from build123d import *

# Parameters (mm, degrees)
SKETCH_1_W                      = 10
SKETCH_1_H                      = 4
EXTRUDE_1_DEPTH                 = 0.6
SKETCH_2_W                      = 6
SKETCH_2_H                      = 2.8
EXTRUDE_2_DEPTH                 = 2.5
FILLET_1_R                      = 1
CUT_EXTRUDE_2_REACH             = 9.134
SKETCH_7_W                      = 0.8
SKETCH_7_H                      = 1
CUT_EXTRUDE_2_DIRECTION_2_DEPTH = 8.134379197
SKETCH_8_W                      = 3.913502977
SKETCH_8_H                      = 4
EXTRUDE_3_DEPTH                 = 0.3
CUT_EXTRUDE_3_REACH             = 9.439
SKETCH_9_W                      = 2
SKETCH_9_H                      = 1
CHAMFER_2_SIZE                  = 0.6
FILLET_2_R                      = 0.3
SKETCH_10_W                     = 0.979037501
SKETCH_10_H                     = 2.8
SKETCH_10_W_2                   = 0.934465476
EXTRUDE_4_DEPTH                 = 1
CHAMFER_3_SIZE                  = 0.3


with BuildPart() as part:
    # 草图1 → 凸台-拉伸1 (new body)
    with BuildSketch(Plane(origin=(0, 0, 0), x_dir=(1, 0, 0), z_dir=(0, 1, 0))):
        with Locations((0.452464262, 0)):
            Rectangle(SKETCH_1_W, SKETCH_1_H)
    extrude(amount=EXTRUDE_1_DEPTH)

    # 草图2 → 凸台-拉伸2 (add)
    with BuildSketch(Plane(origin=(0, 0.6, 0), x_dir=(1, 0, 0), z_dir=(0, 1, 0))):
        with Locations((0.452464262, 0)):
            Rectangle(SKETCH_2_W, SKETCH_2_H)
    extrude(amount=EXTRUDE_2_DEPTH)

    # 圆角1
    fillet_1_edges = [part.edges().sort_by_distance(p)[0] for p in [
        (3.452464262, 1.85, 1.4),
        (3.452464262, 1.85, -1.4),
        (-2.547535738, 1.85, -1.4),
        (-2.547535738, 1.85, 1.4),
        (5.452464262, 0.3, 2),
        (-4.547535738, 0.3, 2),
        (-4.547535738, 0.3, -2),
        (5.452464262, 0.3, -2),
    ]]
    fillet(fillet_1_edges, radius=FILLET_1_R)

    # 草图7 → 切除-拉伸2 (cut, up to next)
    with BuildSketch(Plane.XY.offset(1.4), mode=Mode.PRIVATE) as cut_extrude_2_sk1:
        with Locations((0.474750274, 2.6)):
            Rectangle(SKETCH_7_W, SKETCH_7_H)
    cut_extrude_2_tool1 = extrude(cut_extrude_2_sk1.sketch, amount=-CUT_EXTRUDE_2_REACH, mode=Mode.PRIVATE) & part.part
    add(cut_extrude_2_tool1.solids().sort_by_distance((0.47475, 2.6, 1.4))[0], mode=Mode.SUBTRACT)

    # 草图7 → 切除-拉伸2 direction 2 (cut)
    with BuildSketch(Plane.XY.offset(1.4)):
        with Locations((0.474750274, 2.6)):
            Rectangle(SKETCH_7_W, SKETCH_7_H)
    extrude(amount=CUT_EXTRUDE_2_DIRECTION_2_DEPTH, mode=Mode.SUBTRACT)

    # 草图8 → 凸台-拉伸3 (add)
    with BuildSketch(Plane.XZ):
        with Locations((0.452464261, 0)):
            Rectangle(SKETCH_8_W, SKETCH_8_H)
    extrude(amount=EXTRUDE_3_DEPTH)

    # 草图9 → 切除-拉伸3 (cut, up to next)
    with BuildSketch(Plane(origin=(0, 0, -2), x_dir=(-1, 0, 0), z_dir=(0, 0, -1)), mode=Mode.PRIVATE) as cut_extrude_3_sk1:
        with Locations((-0.474750274, 0.2)):
            Rectangle(SKETCH_9_W, SKETCH_9_H)
    cut_extrude_3_tool1 = extrude(cut_extrude_3_sk1.sketch, amount=-CUT_EXTRUDE_3_REACH, mode=Mode.PRIVATE) & part.part
    add(cut_extrude_3_tool1.solids().sort_by_distance((0.47475, 0.2, -2))[0], mode=Mode.SUBTRACT)

    # 倒角2
    chamfer_2_edges = [part.edges().sort_by_distance(p)[0] for p in [
        (-0.525249726, 0.15, 2),
        (-0.525249726, 0.15, -2),
        (1.474750274, 0.15, -2),
        (1.474750274, 0.15, 2),
    ]]
    chamfer(chamfer_2_edges, length=CHAMFER_2_SIZE)

    # 圆角2
    fillet_2_edges = [part.edges().sort_by_distance(p)[0] for p in [
        (-0.736392732, 3.1, 1.4),
        (-2.547535738, 3.1, 0),
        (3.452464262, 3.1, 0),
        (1.663607268, 3.1, -1.4),
        (3.159571043, 3.1, -1.107106781),
        (-2.25464252, 3.1, -1.107106781),
        (3.159571043, 3.1, 1.107106781),
        (-2.25464252, 3.1, 1.107106781),
        (1.663607268, 3.1, 1.4),
        (-0.736392732, 3.1, -1.4),
    ]]
    fillet(fillet_2_edges, radius=FILLET_2_R)

    # 草图10 → 凸台-拉伸4 (add)
    with BuildSketch(Plane.XZ.offset(0.3)):
        with Locations((-1.014768477, 0)):
            Rectangle(SKETCH_10_W, SKETCH_10_H)
        with Locations((1.941983012, 0)):
            Rectangle(SKETCH_10_W_2, SKETCH_10_H)
    extrude(amount=EXTRUDE_4_DEPTH)

    # 倒角3
    chamfer_3_edges = [part.edges().sort_by_distance(p)[0] for p in [
        (-0.525249726, -0.8, -1.4),
        (-0.525249726, -0.8, 1.4),
        (1.474750274, -0.8, 1.4),
        (1.474750274, -0.8, -1.4),
    ]]
    chamfer(chamfer_3_edges, length=CHAMFER_3_SIZE)


solid = part.part
For this review, take the finished solid that the model builds, in its own axes (mm). A direction names the side the tool comes from. Round coordinates to 2 decimals unless told otherwise and drop trailing zeros. Loops run counter-clockwise (first coordinate to the right, second up) from the corner with the lowest first, then second, coordinate; pieces in that order, holes last. Notation, with made-up numbers: (57.5, -4.75) - (98.5, -4.75) arc R34 ccw to (98.5, 32.25) - close; hole circle Ø9 at (8, 44.5). An arc over 180 degrees is marked (long way). Put each result on its own line as item: value. Start each with the question number.
1. Consider section A-A on y = 2.35. State the section outline as (x, z) points, plus the area to 3 significant figures.
2. Insertion check: P1, Ø0.6, axis at y = -0.5, z = -1, coming from the -X side; P2, Ø1.1, axis at x = 0.5, y = 2, coming from the -Z side; P3, Ø0.9, axis at x = 4, z = -0.5, coming from the -Y side. Each pin has a flat end and moves straight along its axis. Give the tip position at first contact, or say it passes through.
3. For faces 4 (the flat face through (4, 0.6, 0)), 5 (the flat face through (0.4, 1.7, -1.4)), 6 (the flat face through (0.075, 2.6, 0)), 7 (the flat face through (0.4, 1.7, 1.4)), 8 (the flat face through (4, 0, 0)), list the 3-axis set-ups (+Z, -Z, +X, -X, +Y, -Y) from which the entire face can be reached by the end or side of a thin tool; tool diameter is ignored.
4. Consider section D-D on y = 1.55. State the section outline as (x, z) points.
5. For probe 1 along Y at (x, z) = (-3.75, -1); probe 2 along X at (y, z) = (1.65, 0.3); probe 3 along X at (y, z) = (0.3, 1.7), list the stretches that pass through material, from the lowest coordinate up. Write a range as [from, to].
6. Mouldability with a two-part tool opening along X and no side actions: class faces 1 (the flat face through (0, 0.7, 0)), 2 (the flat face through (2.409, -1, 0)), 3 (the cylindrical face through (-2.25, 1.72, 1.11)) as +X half, -X half, draft (parallel to the pull), parting line (faces both ways), or undercut.
7. Consider section C-C on y = 0.3. State the section outline as (x, z) points, plus the area to 3 significant figures.
8. Consider section B-B on z = -0.3. State the section outline as (x, y) points, plus the area to 3 significant figures.
Result sheet:
1. outline: (-2.55, -0.4) arc R1 ccw to (-1.55, -1.4) - (0.07, -1.4) - (0.07, 1.4) - (-1.55, 1.4) arc R1 ccw to (-2.55, 0.4) - close; (0.87, -1.4) - (2.45, -1.4) arc R1 ccw to (3.45, -0.4) - (3.45, 0.4) arc R1 ccw to (2.45, 1.4) - (0.87, 1.4) - close
1. area: 13.7 mm^2
2. P1: x = -1.5
2. P2: z = -1.4
2. P3: y = 0
3. face 4: +X, +Y
3. face 5: -Z, +X, -X, +Y
3. face 6: +Z, -Z, +Y
3. face 7: +Z, +X, -X, +Y
3. face 8: +Z, -Z, +X, -Y
4. outline: (-2.55, -0.4) arc R1 ccw to (-1.55, -1.4) - (2.45, -1.4) arc R1 ccw to (3.45, -0.4) - (3.45, 0.4) arc R1 ccw to (2.45, 1.4) - (-1.55, 1.4) arc R1 ccw to (-2.55, 0.4) - close
5. probe 1: [0, 0.6]
5. probe 2: [-2.55, 3.45]
5. probe 3: [-4.26, -0.83], [1.77, 5.17]
6. face 1: undercut
6. face 2: +X half
6. face 3: -X half
7. outline: (-4.55, -1) arc R1 ccw to (-3.55, -2) - (-1.13, -2) - (-0.53, -1.4) - (-0.53, 1.4) - (-1.13, 2) - (-3.55, 2) arc R1 ccw to (-4.55, 1) - close; (1.47, -1.4) - (2.07, -2) - (4.45, -2) arc R1 ccw to (5.45, -1) - (5.45, 1) arc R1 ccw to (4.45, 2) - (2.07, 2) - (1.47, 1.4) - close
7. area: 30.4 mm^2
8. outline: (-4.55, 0) - (-1.5, 0) - (-1.5, -1.3) - (-0.53, -1.3) - (-0.53, 0.7) - (1.47, 0.7) - (1.47, -1.3) - (2.41, -1.3) - (2.41, 0) - (5.45, 0) - (5.45, 0.6) - (3.45, 0.6) - (3.45, 2.8) arc R0.3 ccw to (3.15, 3.1) - (0.87, 3.1) - (0.87, 2.1) - (0.07, 2.1) - (0.07, 3.1) - (-2.25, 3.1) arc R0.3 ccw to (-2.55, 2.8) - (-2.55, 0.6) - (-4.55, 0.6) - close
8. area: 21.2 mm^2
